Could you check a few things on this model? Use its own coordinates, in mm. Face numbers are marked on the shaded views. A direction names the side the tool comes from. Give positions to 0.01 mm unless a question says otherwise; leave off trailing zeros. Order: outer loops, then holes, each group sorted by start corner. A loop starts at its lowest first (then second) coordinate and runs counter-clockwise, first axis right, second up.
Autodesk Inventor part; units mm, degrees
ref_plane "YZ Plane" through (0, 0, 0) normal (1, 0, 0) x (0, 1, 0)
ref_plane "XZ Plane" through (0, 0, 0) normal (0, 1, 0) x (-1, 0, 0)
ref_plane "XY Plane" through (0, 0, 0) normal (0, 0, 1) x (1, 0, 0)
sketch "Sketch1" plane through (0, 0, 0) normal (0, 0, 1) x (1, 0, 0)
  line L0 (0, 0) -> (15, 0)
  line L1 (15, 0) -> (15, 3)
  line L2 (15, 3) -> (0, 3)
  line L3 (0, 3) -> (0, 0)
  circle A0 centre (0, 2.5) radius 2.5
  point P0 (0, 1.5)
  point P1 (2.4495, 3)
  dimension "d0" = 15
  dimension "d1" = 3
  dimension "d2" = 5
extrude "Extrusion1" add sketch "Sketch1" against normal blind 30
sketch "Sketch2" plane through (0, 0, 0) normal (0, 0, 1) x (1, 0, 0)
  arc A0 (2.4495, 3) -> (0, 0) centre (0, 2.5) ccw
  circle A1 centre (0.0044, 2.5032) radius 2.51
  dimension "d5" = 5.02
extrude "Extrusion2" cut sketch "Sketch2" against normal blind 10
pattern_linear "Rectangular Pattern1" count 2 spacing 20 along (0, 0, -1) of "Extrusion2"
properties part number "Clip1" material "Stainless Steel"
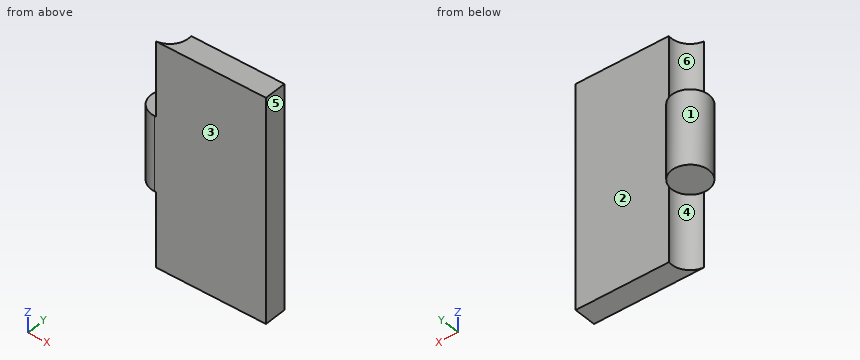
Item 1: For the marked faces 5 and 6, which set-ups out of +Z, -Z, +X, -X, +Y, -Y let a thin tool reach every point of the face, with its end or its side?
Findings:
face 5: +Z, -Z, +X, +Y, -Y
face 6: +Z, -X
Item 2: Imagine slicing it at B-B on x = 13.5. List the corners of the cut face in (y, z) for me.
Findings:
outline: (0, -30) - (3, -30) - (3, 0) - (0, 0) - close
Item 3: For pin 1 (10 mm diameter, centred on x = 6, z = -18, fed in from +Y); pin 2 (1.5 mm diameter, centred on y = 4.5, z = -6, fed in from +X); pin 3 (1.5 mm diameter, centred on x = 0, y = 3.5, fed in from -Z); pin 4 (10 mm diameter, centred on x = 2, z = -3.5, fed in from +Y), each with a flat end and sliding along its axis, tell me the tip position at first contact or that it passes through.
Findings:
pin 1: stops at y = 4.79
pin 2: passes through
pin 3: stops at z = -20
pin 4: stops at y = 3
Item 4: Imagine slicing it at C-C on z = -12.25. List the corners of the cut face in (x, y) for me.
Findings:
outline: (0, 0) - (15, 0) - (15, 3) - (2.45, 3) arc R2.5 ccw (long way) to start
Item 5: Imagine slicing it at A-A on y = 2.5. List the corners of the cut face in (x, z) for me, then the cut area to 3 significant figures.
Findings:
outline: (-2.5, -20) - (2.51, -20) - (2.51, -30) - (15, -30) - (15, 0) - (2.51, 0) - (2.51, -10) - (-2.5, -10) - close
area: 425 mm2
Item 6: Please list where these lines run through material, in increasing order: line 1 along Z through (x, y) = (-0.75, 4.5); line 2 along X through (y, z) = (2.65, -25.75); line 3 along Y through (x, z) = (2.75, -4.5).
Findings:
line 1: z = -20 to -10
line 2: x = 2.51 to 15
line 3: y = 0 to 3
Item 7: Imagine slicing it at D-D on y = 0.6. List the corners of the cut face in (x, z) for me.
Findings:
outline: (-1.62, -20) - (1.64, -20) - (1.64, -30) - (15, -30) - (15, 0) - (1.64, 0) - (1.64, -10) - (-1.62, -10) - close
Item 8: We'd pull the mould along Y, two halves only. Please class the marked faces 1, 2, 3 and 4: +Y half, -Y half, draft (parallel to the pull), parting line (faces both ways), or undercut.
Findings:
face 1: parting line
face 2: +Y half
face 3: -Y half
face 4: undercut
